Design review of the part built by this model. Coordinates are the model's own, in mm. Face numbers are marked on the shaded views. A direction names the side the tool comes from. Give positions to 0.01 mm unless a question says otherwise; leave off trailing zeros. Write each loop counter-clockwise with the first axis right and the second up, starting at its lowest first coordinate (ties: lowest second). Pieces come first, ordered by that corner, then holes.
```python
from build123d import *

# Parameters (mm, degrees)
F1_DEPTH = 25.4
F2_R     = 6.35
F3_DEPTH = 7.62
F4_R     = 5.08
F4_R_2   = 5.588
F4_R_3   = 6.096
F5_DEPTH = 8.89
F7_DEPTH = 6.35


with BuildPart() as f1:
    # F0 (on Top) → F1 (new body)
    with BuildSketch(Plane.XY):
        with BuildLine():
            ThreePointArc((-9.321827, 59.934407), (-17.965589, 42.474951), (-5.735285, 27.310292))
            ThreePointArc((-5.735285, 27.310292), (0, 27.906012), (5.735285, 27.310292))
            ThreePointArc((5.735285, 27.310292), (14.668363, 33.890537), (18.073827, 44.450004))
            ThreePointArc((18.073827, 44.450004), (15.734426, 53.34332), (9.321827, 59.934407))
            Line((9.321827, 59.934407), (-9.321827, 59.934407))
        make_face()
        with BuildLine():
            ThreePointArc((-21.180588, -18.16943), (0, -10.696695), (21.180588, -18.16943))
            ThreePointArc((21.180588, -18.16943), (26.170702, -9.687099), (27.906012, 0))
            ThreePointArc((27.906012, 0), (27.737009, 3.066572), (27.232046, 6.096))
            Line((27.232046, 6.096), (0, 6.096))
            Line((0, 6.096), (-27.232046, 6.096))
            ThreePointArc((-27.232046, 6.096), (-27.076716, -6.752552), (-21.180588, -18.16943))
        make_face()
        with BuildLine():
            ThreePointArc((-21.180588, -18.16943), (-14.566587, -74.898327), (33.753309, -44.450004))
            ThreePointArc((33.753309, -44.450004), (30.448323, -29.883417), (21.180588, -18.16943))
            ThreePointArc((21.180588, -18.16943), (0, -27.906012), (-21.180588, -18.16943))
        make_face()
        with BuildLine():
            ThreePointArc((-21.180588, -18.16943), (0, -27.906012), (21.180588, -18.16943))
            ThreePointArc((21.180588, -18.16943), (0, -10.696695), (-21.180588, -18.16943))
        make_face()
        with BuildLine():
            ThreePointArc((5.735285, 27.310292), (0, 27.906012), (-5.735285, 27.310292))
            ThreePointArc((-5.735285, 27.310292), (0, 26.376177), (5.735285, 27.310292))
        make_face()
        with BuildLine():
            Line((-50.8, 6.096), (-27.232046, 6.096))
            ThreePointArc((-27.232046, 6.096), (-26.296817, 9.339322), (-24.976841, 12.446))
            Line((-24.976841, 12.446), (-50.8, 12.446))
            Line((-50.8, 12.446), (-50.8, 6.096))
        make_face()
        with BuildLine():
            ThreePointArc((24.976841, 12.446), (26.296817, 9.339322), (27.232046, 6.096))
            Line((27.232046, 6.096), (50.8, 6.096))
            Line((50.8, 6.096), (50.8, 12.446))
            Line((50.8, 12.446), (24.976841, 12.446))
        make_face()
        with BuildLine():
            Line((0, 6.096), (27.232046, 6.096))
            ThreePointArc((27.232046, 6.096), (26.296817, 9.339322), (24.976841, 12.446))
            Line((24.976841, 12.446), (0, 12.446))
            Line((0, 12.446), (0, 6.096))
        make_face()
        with BuildLine():
            ThreePointArc((-24.976841, 12.446), (-26.296817, 9.339322), (-27.232046, 6.096))
            Line((-27.232046, 6.096), (0, 6.096))
            Line((0, 6.096), (0, 12.446))
            Line((0, 12.446), (-24.976841, 12.446))
        make_face()
        with BuildLine():
            ThreePointArc((-5.735285, 27.310292), (-17.060055, 22.083932), (-24.976841, 12.446))
            Line((-24.976841, 12.446), (0, 12.446))
            Line((0, 12.446), (24.976841, 12.446))
            ThreePointArc((24.976841, 12.446), (17.060055, 22.083932), (5.735285, 27.310292))
            ThreePointArc((5.735285, 27.310292), (0, 26.376177), (-5.735285, 27.310292))
        make_face()
    extrude(amount=F1_DEPTH)

    # F2 (on face) → F3 (join)
    with BuildSketch(Plane.XY.offset(25.4)):
        with Locations((-8.103234, 47.100332)):
            Circle(F2_R)
        with Locations((7.62, 47.0916)):
            Circle(F2_R)
    extrude(amount=F3_DEPTH)

    # F4 (on face) → F5 (join)
    with BuildSketch(Plane.XY.offset(25.4)):
        with Locations((0, 11.43)):
            Circle(F4_R)
        with Locations((0, -8.72935)):
            Circle(F4_R_2)
        with Locations((0, -25.4)):
            Circle(F4_R_3)
    extrude(amount=F5_DEPTH)

    # F6 (on face) → F7 (join)
    with BuildSketch(Plane.XY.offset(25.4)):
        Polygon((-6.761378, 36.308393), (-4.702554, 33.054311), (6.757731, 33.054311), (8.816555, 36.308393), align=None)
    extrude(amount=F7_DEPTH)


solid = f1.part
```
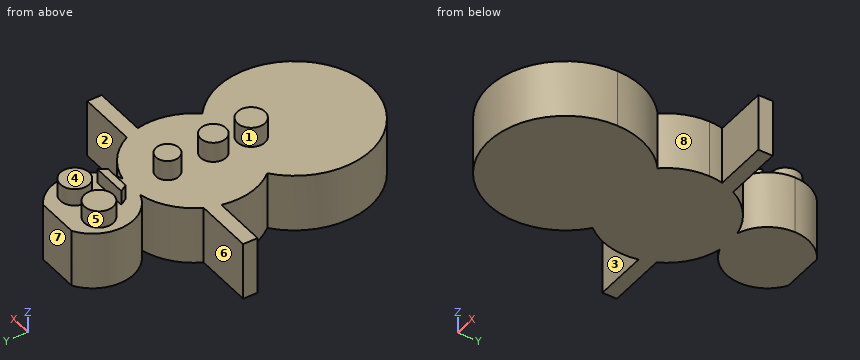
(1) To check wall thickness, follow L1, parallel to Z at x = -4, y = 33.5; L2, parallel to Z at x = -17.5, y = -31.5; L3, parallel to Y at x = -3, z = 31.5. State the ranges of each line that lie inside material, in increasing order.
Resolved:
L1: z = 0 to 31.75
L2: z = 0 to 25.4
L3: y = -30.71 to -20.09, -13.44 to -4.01, 7.33 to 15.53, 33.05 to 36.31, 43.32 to 50.88
(2) Consider section A-A, the plane z = 7. Give the boundary of the cut face in (x, y).
Resolved:
outline: (-50.8, 6.1) - (-27.23, 6.1) arc R27.91 ccw to (-21.18, -18.17) arc R33.75 ccw (long way) to (33.75, -44.45) arc R33.75 ccw to (21.18, -18.17) arc R27.91 ccw to (27.91, 0) arc R27.91 ccw to (27.23, 6.1) - (50.8, 6.1) - (50.8, 12.45) - (24.98, 12.45) arc R27.91 ccw to (5.74, 27.31) arc R18.07 ccw to (18.07, 44.45) arc R18.07 ccw to (9.32, 59.93) - (-9.32, 59.93) arc R18.07 ccw to (-5.74, 27.31) arc R27.91 ccw to (-24.98, 12.45) - (-50.8, 12.45) - close
(3) Tool access review of the marked faces 5, 6, 7 and 8: name each direction out of +Z, -Z, +X, -X, +Y, -Y from which nothing blocks a thin tool from reaching the whole face with its end or side.
Resolved:
face 5: +Z
face 6: +Z, -Z, -X, +Y
face 7: +Z, -Z, +X, -X, +Y
face 8: +Z, -Z, +X
(4) Clearance check with flat-ended pins moving along their axes: P1, Ø12, axis at x = -34, z = 14, coming from the -Y side; P2, Ø3, axis at x = -1.5, z = 29, coming from the -Y side; P3, Ø20.5, axis at x = 37.5, z = 9, coming from the +Y side. State where each tip first meets the part, or that it passes through.
Resolved:
P1: stops at y = -63.3
P2: stops at y = -31.5
P3: stops at y = 12.45
(5) Consider section B-B, the plane x = 11. Give the boundary of the cut face in (y, z).
Resolved:
outline: (-76.36, 0) - (25.65, 0) - (25.65, 25.4) - (-76.36, 25.4) - close; (30.11, 0) - (58.79, 0) - (58.79, 25.4) - (52.47, 25.4) - (52.47, 33.02) - (41.72, 33.02) - (41.72, 25.4) - (30.11, 25.4) - close
(6) Consider section D-D, the plane x = 39.5. Give the boundary of the cut face in (y, z), then the cut area to 3 significant figures.
Resolved:
outline: (6.1, 0) - (12.45, 0) - (12.45, 25.4) - (6.1, 25.4) - close
area: 161 mm2
(7) Consider section C-C, the plane y = -25.4. Give the boundary of the cut face in (x, z), then the cut area to 3 significant figures.
Resolved:
outline: (-27.86, 0) - (27.86, 0) - (27.86, 25.4) - (6.1, 25.4) - (6.1, 34.29) - (-6.1, 34.29) - (-6.1, 25.4) - (-27.86, 25.4) - close
area: 1,520 mm2
(8) Mouldability with a two-part tool opening along Y and no side actions: class the marked faces 1, 2, 3 and 4 as pulls with the +Y half, pulls with the -Y half, needs draft (parallel to the pull), parting line crosses it, or undercut.
Resolved:
face 1: undercut
face 2: pulls with the +Y half
face 3: undercut
face 4: needs draft
